CAD build for the part. Positions are in the model's coordinates, mm. A direction names the side the tool comes from. Coordinates: 2 decimals unless noted, no trailing zeros. Order: outer loops, then holes, each group sorted by start corner. A loop starts at its lowest first (then second) coordinate and runs counter-clockwise, first axis right, second up.
from build123d import *

# Parameters (mm, degrees)
REDONDEO2_R           = 0.5
CROQUIS1_R            = 1
CORTAR_EXTRUIR1_DEPTH = 56.360291205
REDONDEO4_R           = 0.5


with BuildPart() as part:
    # Sketch3 → Revolve1 (revolve)
    with BuildSketch(Plane.XY, mode=Mode.PRIVATE) as revolve1_sk:
        Polygon((7.8, 45.39571665), (7.1, 45.39571665), (8.2, 37.89571665), (7.5, 37.89571665), (8.2, 30.39571665), (7.55, 30.39571665), (7.55, 27.89571665), (11.55, 27.89571665), (11.55, 0), (7.55, 0), (7.55, 25.89571665), (6.1, 25.89571665), (6.1, 52.89571665), (6.9, 52.89571665), align=None)
    revolve(revolve1_sk.sketch.rotate(Axis((0, 70.39571665, 0), (0, -1, 0)), 90), axis=Axis((0, 70.39571665, 0), (0, -1, 0)))

    # Redondeo2
    redondeo2_edges = [part.edges().sort_by_distance(p)[0] for p in [
        (0, 27.89571665, -11.55),
        (0, 0, -11.55),
        (0, 0, -7.55),
    ]]
    fillet(redondeo2_edges, radius=REDONDEO2_R)

    # Croquis1 → Cortar-Extruir1 (cut, through all)
    with BuildSketch(Plane.XY):
        with Locations((0, 13.674991935)):
            Circle(CROQUIS1_R)
    extrude(amount=-CORTAR_EXTRUIR1_DEPTH, mode=Mode.SUBTRACT)

    # Redondeo4
    redondeo4_edges = [part.edges().sort_by_distance(p)[0] for p in [
        (0, 52.89571665, -6.9),
    ]]
    fillet(redondeo4_edges, radius=REDONDEO4_R)


solid = part.part
1) Two-plate mould, pull along X, no slides. Class faces 4 (the conical face through (-2.19, 49.66, 6.95)), 5 (the cylindrical face through (-0.13, 14.666, -9.488)), 6 (the flat face through (7, 27.896, -5)): released by +X, released by -X, zero draft, split by the parting line, or undercut.
2) Slice it at B-B (y = 33). List the corners of the cut face in (x, z).
3) Slice it at A-A (x = 0). Give the number of separate pieces and of enclosed holes in the cut face, plus the area to 3 significant figures.
4) Drill centre lines: probe 1 along X at (y, z) = (13.75, 0); probe 2 along Y at (x, z) = (0, -8.5) (3 decimals); probe 3 along Z at (x, y) = (2, 43.5). Where is each one in solid material? Low to high.
5) Which spindle directions (+Z, -Z, +X, -X, +Y, -Y) get a long thin tool onto all of the face, cutting with end or side? Do faces 1 (the cylindrical face through (-2.27, 13.38, 7.2)), 2 (the cylindrical face through (7.37, 29.13, -1.64)), 3 (the cylindrical face through (3.71, 39.58, -4.84)). Say none if no direction does.
6) Pin check, flat tips, straight feed: P1, Ø1.5, axis at x = 1.5, z = -5, coming from the -Y side; P2, Ø10, axis at x = 8, z = -6, coming from the +Y side; P3, Ø4, axis at x = 6.5, z = 8.5, coming from the +Y side; P4, Ø6, axis at x = 7, y = 18, coming from the -Z side. Stop position of each tip, or through.
Worked out:
1. face 4: split by the parting line
1. face 5: undercut
1. face 6: zero draft
2. outline: circle Ø15.91 at (0, 0); hole circle Ø12.2 at (0, 0)
3. separate pieces: 3
3. enclosed holes: 0
3. area: 296 mm2
4. probe 1: x = -11.55 to -7.55, 7.55 to 11.55
4. probe 2: y = 0 to 12.675, 14.675 to 27.896
4. probe 3: z = -7.1 to -5.76, 5.76 to 7.1
5. face 1: -Y
5. face 2: none
5. face 3: +Y, -Y
6. P1: passes through
6. P2: stops at y = 52.9
6. P3: stops at y = 27.9
6. P4: stops at z = -10.84
